Read the model definition and answer for the solid it produces. Units are mm, in the model's axes. A direction names the side the tool comes from. Give positions to 0.01 mm unless a question says otherwise; leave off trailing zeros. Loops run counter-clockwise (first coordinate to the right, second up) from the corner with the lowest first, then second, coordinate; pieces in that order, holes last. Notation, with made-up numbers: (4.5, 86) -> (37.5, 86) arc R16 cw to (37.5, 99) -> close; hole circle Ø9 at (-0.5, 2). An arc over 180 degrees is marked (long way). One line per item, written item: value. Start each with the question number.
from build123d import *

# Parameters (mm, degrees)
SKETCH_1_W                   = 120
SKETCH_1_H                   = 130
SKETCH_1_W_2                 = 28
SKETCH_1_H_2                 = 45
SM_BASE_FLANGE_1_DEPTH       = 4
SM_START                     = -4
SM_EDGE_FLANGE_1_DEPTH       = 4
SM_EDGE_FLANGE_1_2_OUTLINE_W = 26
SM_EDGE_FLANGE_1_2_OUTLINE_H = 4
SM_EDGE_FLANGE_1_2_DEPTH     = 0.41096
SM_START_2                   = 5
SM_EDGE_FLANGE_1_3_OUTLINE_W = 26
SM_EDGE_FLANGE_1_3_OUTLINE_H = 4
SM_EDGE_FLANGE_1_3_DEPTH     = 20
SM_START_3                   = -13
SM_EDGE_FLANGE_1_4_DEPTH     = 26
SM_EDGE_FLANGE_1_5_DEPTH     = 26
CUT_EXTRUDE_1_DEPTH          = 92.923881554
CUT_EXTRUDE_1_DEPTH_BACK     = 92.923881554
SKETCH_10_R                  = 4.05
SKETCH_12_W                  = 8.2
SKETCH_12_H                  = 8.2
CUT_EXTRUDE_3_DEPTH          = 4
FILLET_1_R                   = 10
SKETCH_11_R                  = 5.1
CUT_EXTRUDE_2_DEPTH          = 4


with BuildPart() as part:
    # Базовая кромка1: sheet metal written as solids
    # Sketch 1 → Базовая кромка1 (new body)
    with BuildSketch(Plane.XY):
        Rectangle(SKETCH_1_W, SKETCH_1_H)
        Rectangle(SKETCH_1_W_2, SKETCH_1_H_2, mode=Mode.SUBTRACT)
    extrude(amount=-SM_BASE_FLANGE_1_DEPTH)

    # Ребро-кромка1: read off the stored shape, not the designer's step
    # Ребро-кромка1 outline → Ребро-кромка1 (cut)
    with BuildSketch(Plane.XY.offset(SM_START)):
        with BuildLine():
            ThreePointArc((-13, 31.6), (-13.5, 32.1), (-14, 31.6))
            Line((-14, 31.6), (-14, 22.5))
            Line((-14, 22.5), (-13, 22.5))
            Line((-13, 22.5), (-13, 31.6))
        make_face()
        with BuildLine():
            Line((-13, -22.5), (-14, -22.5))
            Line((-14, -22.5), (-14, -31.6))
            ThreePointArc((-14, -31.6), (-13.5, -32.1), (-13, -31.6))
            Line((-13, -31.6), (-13, -22.5))
        make_face()
        with BuildLine():
            Line((13, 31.6), (13, 22.5))
            Line((13, 22.5), (14, 22.5))
            Line((14, 22.5), (14, 31.6))
            ThreePointArc((14, 31.6), (13.5, 32.1), (13, 31.6))
        make_face()
        with BuildLine():
            Line((14, -22.5), (13, -22.5))
            Line((13, -22.5), (13, -31.6))
            ThreePointArc((13, -31.6), (13.5, -32.1), (14, -31.6))
            Line((14, -31.6), (14, -22.5))
        make_face()
    extrude(amount=SM_EDGE_FLANGE_1_DEPTH, mode=Mode.SUBTRACT)

    # Sm Edge Flange 1 2 outline → Sm Edge Flange 1 2 (cut)
    with BuildSketch(Plane.XY.offset(SM_START)):
        with Locations((0, 24.5)):
            Rectangle(SM_EDGE_FLANGE_1_2_OUTLINE_W, SM_EDGE_FLANGE_1_2_OUTLINE_H)
        with Locations((0, -24.5)):
            Rectangle(SM_EDGE_FLANGE_1_2_OUTLINE_W, SM_EDGE_FLANGE_1_2_OUTLINE_H)
    extrude(amount=SM_EDGE_FLANGE_1_2_DEPTH, mode=Mode.SUBTRACT)

    # Sm Edge Flange 1 4 outline → Sm Edge Flange 1 4 (cut)
    with BuildSketch(Plane.YZ.offset(SM_START_3)):
        with BuildLine():
            ThreePointArc((31.5, -4), (27.257359313, -2.937253933), (24.016685226, 0))
            Line((24.016685226, 0), (22.5, 0))
            Line((22.5, 0), (22.5, -3.58904))
            Line((22.5, -3.58904), (26.5, -3.58904))
            Line((26.5, -3.58904), (26.5, -4))
            Line((26.5, -4), (31.5, -4))
        make_face()
        with BuildLine():
            Line((-22.5, -3.58904), (-22.5, 0))
            Line((-22.5, 0), (-24.016685226, 0))
            ThreePointArc((-24.016685226, 0), (-27.257359313, -2.937253933), (-31.5, -4))
            Line((-31.5, -4), (-26.5, -4))
            Line((-26.5, -4), (-26.5, -3.58904))
            Line((-26.5, -3.58904), (-22.5, -3.58904))
        make_face()
    extrude(amount=SM_EDGE_FLANGE_1_4_DEPTH, mode=Mode.SUBTRACT)



with BuildPart() as body_2:
    # Sm Edge Flange 1 3 outline → Sm Edge Flange 1 3 (new body)
    with BuildSketch(Plane.XY.offset(SM_START_2)):
        with Locations((0, 24.5)):
            Rectangle(SM_EDGE_FLANGE_1_3_OUTLINE_W, SM_EDGE_FLANGE_1_3_OUTLINE_H)
        with Locations((0, -24.5)):
            Rectangle(SM_EDGE_FLANGE_1_3_OUTLINE_W, SM_EDGE_FLANGE_1_3_OUTLINE_H)
    extrude(amount=SM_EDGE_FLANGE_1_3_DEPTH)


with BuildPart() as part_1:
    add(part.part)

    add(body_2.part)  # Sm Edge Flange 1 5 merges body 2
    # Sm Edge Flange 1 5 outline → Sm Edge Flange 1 5 (add)
    with BuildSketch(Plane.YZ.offset(SM_START_3)):
        with BuildLine():
            Line((26.5, 5), (22.5, 5))
            ThreePointArc((22.5, 5), (22.88751392, 2.38751392), (24.016685226, 0))
            Line((24.016685226, 0), (31.5, 0))
            ThreePointArc((31.5, 0), (27.964466094, 1.464466094), (26.5, 5))
        make_face()
        with BuildLine():
            Line((-31.5, 0), (-24.016685226, 0))
            ThreePointArc((-24.016685226, 0), (-22.88751392, 2.38751392), (-22.5, 5))
            Line((-22.5, 5), (-26.5, 5))
            ThreePointArc((-26.5, 5), (-27.964466094, 1.464466094), (-31.5, 0))
        make_face()
    extrude(amount=SM_EDGE_FLANGE_1_5_DEPTH)

    # Эскиз10 → Вырез-Вытянуть1 (cut, two sides: drawn at the far end of the back side and taken through both)
    with BuildSketch(Plane(origin=(0, 0, 0), x_dir=(1, 0, 0), z_dir=(0, 1, 0)).offset(-CUT_EXTRUDE_1_DEPTH_BACK)):
        with Locations(Location((0, -17, 0), (0, 0, 90))):
            Circle(SKETCH_10_R)
    extrude(amount=CUT_EXTRUDE_1_DEPTH + CUT_EXTRUDE_1_DEPTH_BACK, mode=Mode.SUBTRACT)

    # Эскиз12 → Вырез-Вытянуть3 (cut)
    with BuildSketch(Plane(origin=(0, 26.5, 0), x_dir=(1, 0, 0), z_dir=(0, 1, 0))):
        with Locations((0, -17)):
            Rectangle(SKETCH_12_W, SKETCH_12_H)
    extrude(amount=-CUT_EXTRUDE_3_DEPTH, mode=Mode.SUBTRACT)

    # Скругление1
    fillet_1_edges = [part_1.edges().sort_by_distance(p)[0] for p in [
        (13, -24.5, 25),
        (-13, -24.5, 25),
        (-60, 65, -2),
        (60, 65, -2),
        (60, -65, -2),
        (-60, -65, -2),
        (-13, 24.5, 25),
        (13, 24.5, 25),
    ]]
    fillet(fillet_1_edges, radius=FILLET_1_R)

    # Эскиз11 → Вырез-Вытянуть2 (cut)
    with BuildSketch(Plane.XY):
        with Locations((-45, 50)):
            Circle(SKETCH_11_R)
        with Locations((45, 50)):
            Circle(SKETCH_11_R)
        with Locations((-45, -50)):
            Circle(SKETCH_11_R)
        with Locations((45, -50)):
            Circle(SKETCH_11_R)
    extrude(amount=-CUT_EXTRUDE_2_DEPTH, mode=Mode.SUBTRACT)


solid = part_1.part
Item 1: Section A-A, the plane x = 11 is taken. Determine the outline of the cut face in (y, z).
Item 2: For faces 1 (the flat face through (-0.2, -26.5, 12.6)), 2 (the cylindrical face through (41.2, 53.4, -2)), 3 (the flat face through (-4.1, 25, 17)), determine the directions among +Z, -Z, +X, -X, +Y, -Y from which every point of the face is accessible in a straight line to the end or side of a thin tool.
Item 3: Section C-C, the plane x = -45 is taken. Determine the outline of the cut face in (y, z).
Item 4: Section D-D, the plane y = 13 is taken. Determine the outline of the cut face in (x, z).
Item 5: Determine the mould class of faces 4 (the cylindrical face through (10.15, 24.53, 21.99)), 5 (the cylindrical face through (-57.15, 61.99, -2.03)), 6 (the cylindrical face through (-50.095, -49.776, -1.972)) for opening direction Y: pulls with the +Y half, pulls with the -Y half, needs draft (parallel to the pull), parting line crosses it, or undercut.
Item 6: Consider L1, parallel to Y at x = 45, z = -2.65; L2, parallel to Y at x = 7.5, z = 10.5; L3, parallel to X at y = 25.5, z = 12.25. Determine where each line is inside the solid, lowest interval first. Write a range as [from, to].
Item 7: Flat-ended cylindrical pins translate along their axes: pin 1 (2.5 mm diameter, centred on y = -27, z = 7.5, fed in from -X); pin 2 (2 mm diameter, centred on x = -1, y = 25.5, fed in from -Z); pin 3 (13.5 mm diameter, centred on x = -45, y = 50, fed in from +Z). Find the tip coordinate at first contact, or state that the pin passes through.
Item 8: Section B-B, the plane y = 50 is taken. Determine the outline of the cut face in (x, z).
Computed values:
1. outline: (-65, -4) -> (-31.5, -4) arc R9 ccw to (-22.5, 5) -> (-22.5, 21) -> (-26.5, 21) -> (-26.5, 5) arc R5 cw to (-31.5, 0) -> (-65, 0) -> close; (22.5, 5) arc R9 ccw to (31.5, -4) -> (65, -4) -> (65, 0) -> (31.5, 0) arc R5 cw to (26.5, 5) -> (26.5, 21) -> (22.5, 21) -> close
2. face 1: +Z, +X, -X, -Y
2. face 2: +Z, -Z
2. face 3: +Y
3. outline: (-65, -4) -> (-55.1, -4) -> (-55.1, 0) -> (-65, 0) -> close; (-44.9, -4) -> (44.9, -4) -> (44.9, 0) -> (-44.9, 0) -> close; (55.1, -4) -> (65, -4) -> (65, 0) -> (55.1, 0) -> close
4. outline: (-60, -4) -> (-14, -4) -> (-14, 0) -> (-60, 0) -> close; (14, -4) -> (60, -4) -> (60, 0) -> (14, 0) -> close
5. face 4: needs draft
5. face 5: pulls with the +Y half
5. face 6: undercut
6. L1: [-65, -55.1], [-44.9, 44.9], [55.1, 65]
6. L2: [-26.5, -22.5], [22.5, 26.5]
6. L3: [-13, 13]
7. pin 1: x = -13
7. pin 2: z = -2.48
7. pin 3: z = 0
8. outline: (-60, -4) -> (-50.1, -4) -> (-50.1, 0) -> (-60, 0) -> close; (-39.9, -4) -> (39.9, -4) -> (39.9, 0) -> (-39.9, 0) -> close; (50.1, -4) -> (60, -4) -> (60, 0) -> (50.1, 0) -> close
